Here's how the part is built. I have some questions about the finished solid (model axes, mm). A direction names the side the tool comes from. Coordinates: 2 decimals unless noted, no trailing zeros. Write each loop counter-clockwise with the first axis right and the second up, starting at its lowest first coordinate (ties: lowest second). Pieces come first, ordered by that corner, then holes. Notation, with made-up numbers: (-39, 6) - (7, 6) arc R30 cw to (7, 37) - close; hole circle Ø3 at (16, 3). An arc over 180 degrees is marked (long way). Answer in a Markdown table with one row per item. Add a question column.
Item 1: If I drill on probe 1 along X at (y, z) = (653, -485); probe 2 along Z at (x, y) = (618, 464); probe 3 along Y at (x, z) = (402, -207), over which ranges is the centre line in solid material (lowest first)? Write a range as from..to.
Item 2: I'm going to push flat-ended pins straight in: pin 1 (1.5 mm diameter, centred on x = 788.5, y = 850, fed in from -Z); pin 2 (21 mm diameter, centred on x = 1561.5, z = -183, fed in from -Y); pin 3 (1 mm diameter, centred on x = 1583, z = -307, fed in from +Y). Where does each tip first touch, or does it pass through?
Item 3: Imagine slicing it at C-C (x = 1408.5). Please give me the cut outline in (y, z), plus the area to 3 significant figures.
Item 4: Imagine slicing it at D-D (y = 877.5). Please give me the cut outline in (x, z).
Item 5: Imagine slicing it at A-A (z = -432). Please give me the cut outline in (x, y), plus the area to 3 significant figures.
Item 6: Which directions (+Z, -Z, +X, -X, +Y, -Y) give clear straight access to the entire face, cutting with the end or side of a thin tool? Please do faces 1 (the face through (470, 313, -345)), 2 (the face through (1565, 480, -355)), 3 (the face through (1600, 313, -345)), 4 (the face through (400, 313, -345)), 5 (the face through (1565, 850, -345)).
Item 7: Imagine slicing it at B-B (y = 616). Please give me the cut outline in (x, z).
Item 8: We'd pull the mould along Y, two halves only. Please class faces 6 (the face through (1530, 683, -345)), 7 (the face through (435, 520, -355)), 8 (the face through (435, 480, -355)), 9 (the face through (435, 150, -345)): +Y half, -Y half, draft (parallel to the pull), parting line (faces both ways), or undercut.
from build123d import *

# Parameters (mm, degrees)
F0_W     = 2000
F0_H     = 1000
F1_DEPTH = 70
F2_W     = 70
F2_H     = 700
F3_DEPTH = 700
F4_W     = 40
F4_H     = 700
F5_DEPTH = 1600.001


with BuildPart() as f1:
    # F0 (on Top) → F1 (new body)
    with BuildSketch(Plane.XY):
        with Locations((1000, 500)):
            Rectangle(F0_W, F0_H)
    extrude(amount=F1_DEPTH)

    # F2 (on Top) → F3 (join)
    with BuildSketch(Plane.XY):
        with Locations((435, 500)):
            Rectangle(F2_W, F2_H)
        with Locations((1565, 500)):
            Rectangle(F2_W, F2_H)
    extrude(amount=-F3_DEPTH)

    # F4 (on face) → F5 (cut, through all)
    with BuildSketch(Plane.YZ.offset(1600)):
        with Locations((500, -350)):
            Rectangle(F4_W, F4_H)
    extrude(amount=-F5_DEPTH, mode=Mode.SUBTRACT)


solid = f1.part
Here are the results:
| question | item | result |
|---|---|---|
| 1 | probe 1 | x = 400..470, 1530..1600 |
| 1 | probe 2 | z = 0..70 |
| 1 | probe 3 | y = 150..480, 520..850 |
| 2 | pin 1 | stops at z = 0 |
| 2 | pin 2 | stops at y = 150 |
| 2 | pin 3 | stops at y = 850 |
| 3 | outline | (0, 0) - (1000, 0) - (1000, 70) - (0, 70) - close |
| 3 | area | 70,000 mm2 |
| 4 | outline | (0, 0) - (2000, 0) - (2000, 70) - (0, 70) - close |
| 5 | outline | (400, 150) - (470, 150) - (470, 480) - (400, 480) - close; (400, 520) - (470, 520) - (470, 850) - (400, 850) - close; (1530, 150) - (1600, 150) - (1600, 480) - (1530, 480) - close; (1530, 520) - (1600, 520) - (1600, 850) - (1530, 850) - close |
| 5 | area | 92,400 mm2 |
| 6 | face 1 | -Z, +Y, -Y |
| 6 | face 2 | -Z, +X, -X |
| 6 | face 3 | -Z, +X, +Y, -Y |
| 6 | face 4 | -Z, -X, +Y, -Y |
| 6 | face 5 | -Z, +X, -X, +Y |
| 7 | outline | (0, 0) - (400, 0) - (400, -700) - (470, -700) - (470, 0) - (1530, 0) - (1530, -700) - (1600, -700) - (1600, 0) - (2000, 0) - (2000, 70) - (0, 70) - close |
| 8 | face 6 | draft |
| 8 | face 7 | undercut |
| 8 | face 8 | undercut |
| 8 | face 9 | -Y half |
